Print and shaded views of the part. All mm, measured from the part's lowest x, y and z. A direction names the side the tool comes from. Round coordinates to 2 decimals unless told otherwise and drop trailing zeros. Loops run counter-clockwise (first coordinate to the right, second up) from the corner with the lowest first, then second, coordinate; pieces in that order, holes last. Notation, with made-up numbers: M -25,-3.75 L -10,-3.75 A22 cw -10,24.25 Z; hole C -7,59 d1. An arc over 180 degrees is marked long. One line per item, written item: value. Start each with the question number.
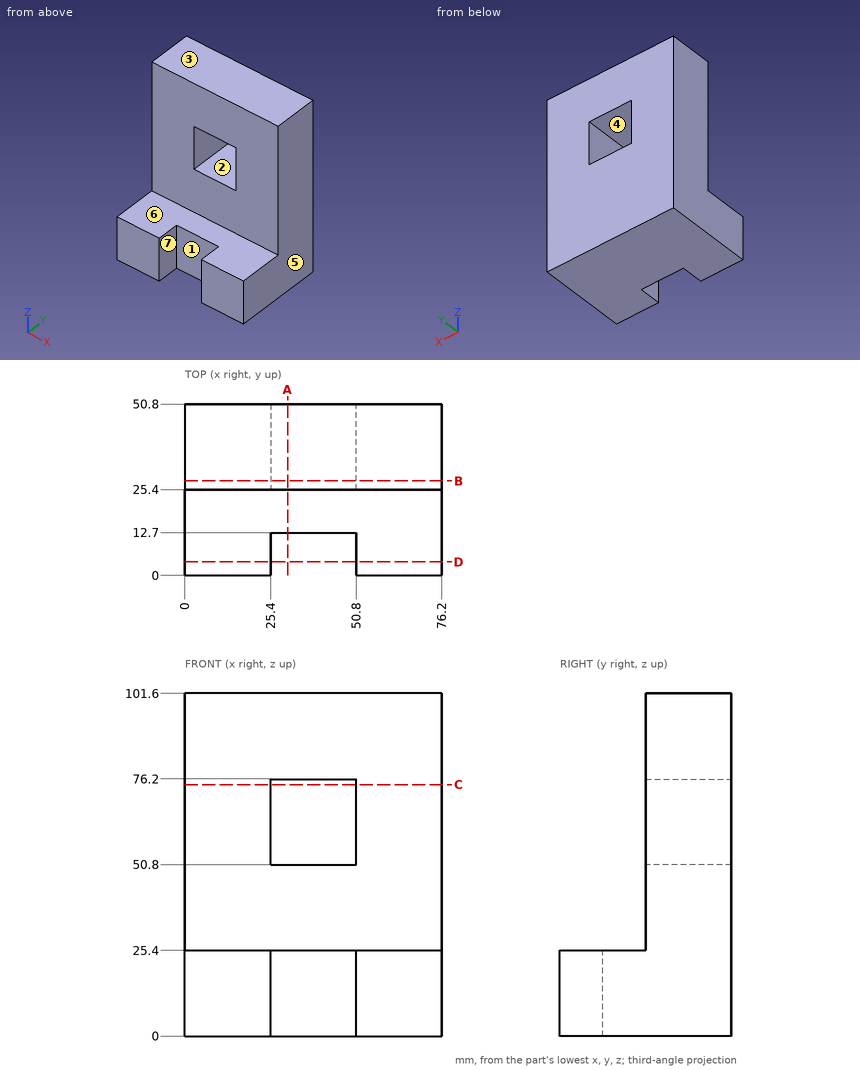
(1) Probe L1, parallel to X at y = 27.5, z = 73; L2, parallel to Z at x = 33, y = 48.5; L3, parallel to Z at x = 26, y = 17. List the from-to ranges inside material, lowest first.
(2) Which spindle directions (+Z, -Z, +X, -X, +Y, -Y) get a long thin tool onto all of the face, cutting with end or side? Do the marked faces 4, 5, 6 and 7. Say none if no direction does.
(3) Slice it at B-B, the plane y = 28. List the corners of the cut face in (x, z).
(4) Flat gauge pin, fed straight in: P1, Ø12.5, axis at x = 23.5, y = 15, coming from the +Z side. Where does the tip first touch, or does it go through?
(5) Slice it at D-D, the plane y = 4. List the corners of the cut face in (x, z), and give its area (3 significant figures).
(6) Mould opens along Z. For the marked faces 1, 2 and 3 say: pulls with the +Z half, pulls with the -Z half, needs draft (parallel to the pull), parting line crosses it, or undercut.
(7) Slice it at C-C, the plane z = 74.5. List the corners of the cut face in (x, y).
(8) Slice it at A-A, the plane x = 30.5. List the corners of the cut face in (y, z).
Check result:
1. L1: x = 0 to 25.4, 50.8 to 76.2
1. L2: z = 0 to 50.8, 76.2 to 101.6
1. L3: z = 0 to 25.4
2. face 4: +Y, -Y
2. face 5: +Z, -Z, +X, +Y, -Y
2. face 6: +Z, +X, -X, -Y
2. face 7: +Z, -Z, -Y
3. outline: M 0,0 L 76.2,0 L 76.2,101.6 L 0,101.6 Z; hole M 25.4,50.8 L 50.8,50.8 L 50.8,76.2 L 25.4,76.2 Z
4. P1: stops at z = 25.4
5. outline: M 0,0 L 25.4,0 L 25.4,25.4 L 0,25.4 Z; M 50.8,0 L 76.2,0 L 76.2,25.4 L 50.8,25.4 Z
5. area: 1,290 mm^2
6. face 1: needs draft
6. face 2: undercut
6. face 3: pulls with the +Z half
7. outline: M 0,25.4 L 25.4,25.4 L 25.4,50.8 L 0,50.8 Z; M 50.8,25.4 L 76.2,25.4 L 76.2,50.8 L 50.8,50.8 Z
8. outline: M 12.7,0 L 50.8,0 L 50.8,50.8 L 25.4,50.8 L 25.4,25.4 L 12.7,25.4 Z; M 25.4,76.2 L 50.8,76.2 L 50.8,101.6 L 25.4,101.6 Z
